Input: part model. Units: mm. Frame: model coordinates. Face numbers are marked on the shaded views. A direction names the side the tool comes from. Give positions to 0.01 mm unless a question says otherwise; leave off trailing zeros. Loops run counter-clockwise (first coordinate to the right, second up) from the corner with the lowest first, then second, coordinate; pieces in that order, holes last. Notation, with made-up numbers: M -16,86 L 12,86 A20 ccw 12,123 Z; hole C -35.5,42 d1. An arc over 180 degrees is marked long. Answer as a JSON object with one key per item and string values. Group by question number.
1) Section query B-B on z = 0. Return loops of the section in (x, y) (3 decimals).
2) Draft query along Z for the marked faces 1, 2 and 3. Return one class per face: +Z half, -Z half, draft (parallel to the pull), parting line (faces both ways), or undercut.
3) Access query for the marked faces 4, 5 and 6. Directions: +Z, -Z, +X, -X, +Y, -Y. A direction counts if a zero-diameter tool reaches every point of the face in a straight line with its end or side. Return the directions, or none.
4) Ray query, L1, parallel to X at y = 25, z = 0 (3 decimals); L2, parallel to Z at x = 0, y = 7; L3, parallel to X at y = 26.5, z = 0 (3 decimals). Return the intervals inside material, ascending.
5) Section query A-A on x = 0. Return loops of the section in (y, z) (3 decimals).
6) First-contact query: P1, Ø1, axis at x = -3, y = 16.5, coming from the -Z side; P2, Ø4, axis at x = 0, z = 0, coming from the -Y side; P3, Ø4, axis at x = 4, y = 30, coming from the +Z side; P4, Ø4, axis at x = -1, z = -1.5, coming from the -Y side. Flat tips, straight axial feed; report the tip coordinate or a pass-through.
7) Section query D-D on x = -3.75. Return loops of the section in (y, z).
8) Section query C-C on y = 18. Return loops of the section in (x, z) (3 decimals).
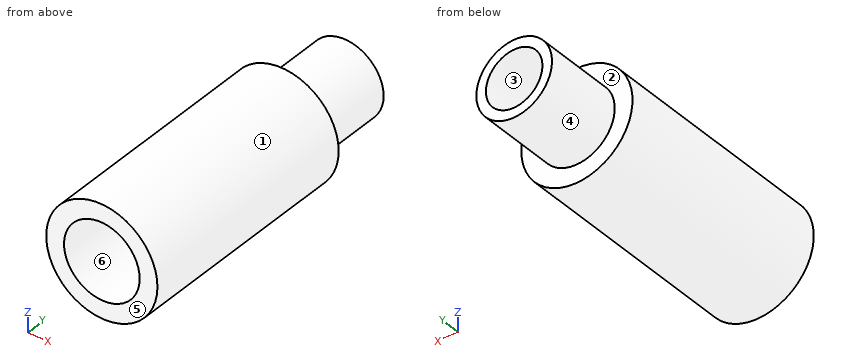
from build123d import *

# Parameters (mm, degrees)
SKETCH1_R           = 6.25
SKETCH1_R_2         = 3.175
BOSS_EXTRUDE1_DEPTH = 35
SKETCH2_OUTSIDE_W   = 22.342
SKETCH2_OUTSIDE_H   = 22.342
SKETCH2_OUTSIDE_R   = 4.25
CUT_EXTRUDE1_DEPTH  = 9
SKETCH3_R           = 4.25
CUT_EXTRUDE2_DEPTH  = 9


with BuildPart() as part:
    # Sketch1 → Boss-Extrude1 (new body)
    with BuildSketch(Plane(origin=(0, 0, 0), x_dir=(1, 0, 0), z_dir=(0, 1, 0))):
        Circle(SKETCH1_R)
        Circle(SKETCH1_R_2, mode=Mode.SUBTRACT)
    extrude(amount=BOSS_EXTRUDE1_DEPTH)

    # Sketch2 outside → Cut-Extrude1 (cut)
    with BuildSketch(Plane(origin=(0, 35, 0), x_dir=(1, 0, 0), z_dir=(0, 1, 0))):
        Rectangle(SKETCH2_OUTSIDE_W, SKETCH2_OUTSIDE_H)
        Circle(SKETCH2_OUTSIDE_R, mode=Mode.SUBTRACT)
    extrude(amount=-CUT_EXTRUDE1_DEPTH, mode=Mode.SUBTRACT)

    # Sketch3 → Cut-Extrude2 (cut)
    with BuildSketch(Plane.XZ):
        Circle(SKETCH3_R)
    extrude(amount=-CUT_EXTRUDE2_DEPTH, mode=Mode.SUBTRACT)


solid = part.part
Output:
{
 "1": {"outline": "M -6.25,0 L -4.25,0 L -4.25,9 L -3.175,9 L -3.175,35 L -4.25,35 L -4.25,26 L -6.25,26 Z; M 3.175,9 L 4.25,9 L 4.25,0 L 6.25,0 L 6.25,26 L 4.25,26 L 4.25,35 L 3.175,35 Z"},
 "2": {"face 1": "parting line", "face 2": "draft", "face 3": "undercut"},
 "3": {"face 4": "+Y", "face 5": "+Z, -Z, +X, -X, -Y", "face 6": "-Y"},
 "4": {"L1": "x = -6.25 to -3.175, 3.175 to 6.25", "L2": "z = -6.25 to -4.25, 4.25 to 6.25", "L3": "x = -4.25 to -3.175, 3.175 to 4.25"},
 "5": {"outline": "M 0,-6.25 L 26,-6.25 L 26,-4.25 L 35,-4.25 L 35,-3.175 L 9,-3.175 L 9,-4.25 L 0,-4.25 Z; M 0,4.25 L 9,4.25 L 9,3.175 L 35,3.175 L 35,4.25 L 26,4.25 L 26,6.25 L 0,6.25 Z"},
 "6": {"P1": "stops at z = -5.73", "P2": "passes through", "P3": "stops at z = 3.75", "P4": "stops at y = 9"},
 "7": {"outline": "M 0,-5 L 26,-5 L 26,-2 L 35,-2 L 35,2 L 26,2 L 26,5 L 0,5 L 0,2 L 9,2 L 9,-2 L 0,-2 Z"},
 "8": {"outline": "C 0,0 d12.5; hole C 0,0 d6.35"}
}
